For this review, take the finished solid that the model builds, in its own axes (mm). Round coordinates to 2 decimals unless told otherwise and drop trailing zeros. Loops run counter-clockwise (first coordinate to the right, second up) from the corner with the lowest first, then second, coordinate; pieces in that order, holes last.
```python
from build123d import *

# Parameters (mm, degrees)
SKETCH1_R               = 3
BOSS_EXTRUDE1_DEPTH     = 80
SKETCH2_R               = 6.35
BOSS_EXTRUDE2_DEPTH     = 600
SKETCH3_W               = 12.7
SKETCH3_H               = 521.5
CUT_EXTRUDE1_DEPTH      = 7
CUT_EXTRUDE1_DEPTH_BACK = 7


with BuildPart() as part:
    # Sketch1 → Boss-Extrude1 (new body)
    with BuildSketch(Plane(origin=(0, 0, 0), x_dir=(1, 0, 0), z_dir=(0, 1, 0))):
        Circle(SKETCH1_R)
    extrude(amount=BOSS_EXTRUDE1_DEPTH)

    # Sketch2 → Boss-Extrude2 (add)
    with BuildSketch(Plane(origin=(0, 80, 0), x_dir=(1, 0, 0), z_dir=(0, 1, 0))):
        Circle(SKETCH2_R)
    extrude(amount=-BOSS_EXTRUDE2_DEPTH)

    # Sketch3 → Cut-Extrude1 (cut, two sides)
    with BuildSketch(Plane(origin=(0, 0, 0), x_dir=(0, 0, -1), z_dir=(1, 0, 0))) as cut_extrude1_sk:
        with Locations((0, -259.25)):
            Rectangle(SKETCH3_W, SKETCH3_H)
    extrude(amount=CUT_EXTRUDE1_DEPTH, mode=Mode.SUBTRACT)
    extrude(cut_extrude1_sk.sketch, amount=-CUT_EXTRUDE1_DEPTH_BACK, mode=Mode.SUBTRACT)


solid = part.part
```
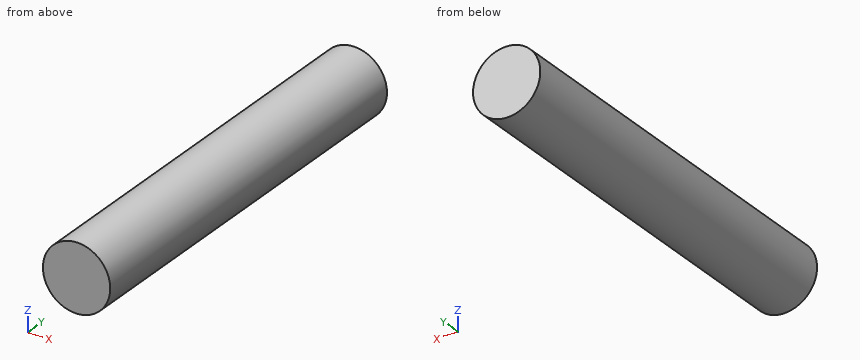
(1) Add section C-C (z = 2). Give the boundary of the cut face in (x, y), plus the area to 3 significant figures.
(2) Add section B-B (x = -2). Give the boundary of the cut face in (y, z).
(3) For L1, parallel to X at y = 69, z = -0.25; L2, parallel to Z at x = -1.75, y = 35.5, list the stretches that pass through material, from the lowest coordinate up.
(4) Add section A-A (y = 51). Give the boundary of the cut face in (x, z).
(5) Insertion check: pin 1 Ø1 at (x, y) = (-2, 24.5) entering from -Z; pin 2 Ø4 at (y, z) = (21.5, 3) entering from -X. Each pin has a flat end and moves straight along its axis. Give the tip position at first contact, or say it passes through.
Outcome:
1. outline: (-6.03, 1.5) - (6.03, 1.5) - (6.03, 80) - (-6.03, 80) - close
1. area: 946 mm2
2. outline: (1.5, -6.03) - (80, -6.03) - (80, 6.03) - (1.5, 6.03) - close
3. L1: x = -6.35 to 6.35
3. L2: z = -6.1 to 6.1
4. outline: circle Ø12.7 at (0, 0)
5. pin 1: stops at z = -6.17
5. pin 2: stops at x = -6.27
